```python
from build123d import *

# Parameters (mm, degrees)
F0_W     = 60
F0_H     = 60
F1_DEPTH = 32
F2_W     = 18
F2_H     = 20
F3_DEPTH = 60.001
F4_W     = 35
F4_H     = 10
F5_DEPTH = 60.001
F6_R     = 17.5
F6_R_2   = 10
F7_DEPTH = 64


with BuildPart() as f1:
    # F0 (on Top) → F1 (new body)
    with BuildSketch(Plane.XY):
        with Locations((0.728403, 0.219683)):
            Rectangle(F0_W, F0_H)
    extrude(amount=F1_DEPTH)

    # F2 (on face) → F3 (cut, through all)
    with BuildSketch(Plane.XZ.offset(29.780317)):
        with Locations((0.728403, 10)):
            Rectangle(F2_W, F2_H)
    extrude(amount=-F3_DEPTH, mode=Mode.SUBTRACT)

    # F4 (on face) → F5 (cut, through all)
    with BuildSketch(Plane.YZ.offset(30.728403)):
        with Locations((0.219683, 5)):
            Rectangle(F4_W, F4_H)
    extrude(amount=-F5_DEPTH, mode=Mode.SUBTRACT)

    # F6 (on face) → F7 (join)
    with BuildSketch(Plane.XY.offset(32)):
        Circle(F6_R)
        Circle(F6_R_2, mode=Mode.SUBTRACT)
    extrude(amount=F7_DEPTH)


solid = f1.part
```
Geometry: final body of the model. Coordinates: model frame, mm. A direction names the side the tool comes from. Coordinates: 2 decimals unless noted, no trailing zeros. Order: outer loops, then holes, each group sorted by start corner. A loop starts at its lowest first (then second) coordinate and runs counter-clockwise, first axis right, second up. Notation, with made-up numbers: (53.5, 85) -> (103.5, 85) arc R24 ccw to (103.5, 118) -> close; hole circle Ø3 at (-8.75, 22). An arc over 180 degrees is marked (long way). Use CSV: the item, a comma, the result in double quotes.
1) Access query for faces 5 (the flat face through (9.728, 0, 12)), 6 (the flat face through (0, 0, 32)), 7 (the flat face through (-19, 0, 10)), 8 (the flat face through (0, 30.22, 23)), 9 (the flat face through (30.728, 0, 19)). Directions: +Z, -Z, +X, -X, +Y, -Y. A direction counts if a zero-diameter tool reaches every point of the face in a straight line with its end or side. Return the directions, or none.
Findings:
face 5,"-Z, +Y, -Y"
face 6,"+Z"
face 7,"-Z, +X, -X"
face 8,"+Z, -Z, +X, -X, +Y"
face 9,"+Z, -Z, +X, +Y, -Y"
2) Section A-A on x = 0. Output: boundary loops of the cut face in (y, z).
Findings:
outline,"(-29.78, 20) -> (30.22, 20) -> (30.22, 32) -> (17.5, 32) -> (17.5, 96) -> (10, 96) -> (10, 32) -> (-10, 32) -> (-10, 96) -> (-17.5, 96) -> (-17.5, 32) -> (-29.78, 32) -> close"
3) Mould query, pull axis X, two halves, no side actions, for faces 1 (the flat face through (-29.272, 0, 19)), 2 (the cylindrical face through (-2.17, -9.76, 63.55)), 3 (the flat face through (-19, 24, 0)), 4 (the flat face through (1, 0, 20)). Classes: +X half, -X half, draft (parallel to the pull), parting line (faces both ways), or undercut.
Findings:
face 1,"-X half"
face 2,"undercut"
face 3,"draft"
face 4,"undercut"
4) Section C-C on z = 44.5. Output: boundary loops of the cut face in (x, y), then the cut area to 3 significant figures.
Findings:
outline,"circle Ø35 at (0, 0); hole circle Ø20 at (0, 0)"
area,"648 mm^2"
5) Line query: line 1 (Y direction, x = 0, z = 50); line 2 (X direction, y = -0.5, z = 11.5); line 3 (Z direction, x = -21, y = 13). Output: solid intervals per line, ascending.
Findings:
line 1,"y = -17.5 to -10, 10 to 17.5"
line 2,"x = -29.27 to -8.27, 9.73 to 30.73"
line 3,"z = 10 to 32"
6) Pin query (flat end, axial travel): pin 1 Ø5 at (x, z) = (-8, 40.5) entering from +Y; pin 2 Ø10.5 at (x, y) = (-22.5, -1.5) entering from -Z; pin 3 Ø3 at (x, y) = (-14.5, -23.5) entering from +Z. Return the tip coordinate at first contact, or that it passes through.
Findings:
pin 1,"stops at y = 16.61"
pin 2,"stops at z = 10"
pin 3,"stops at z = 32"
7) Section D-D on x = -20. Output: boundary loops of the cut face in (y, z).
Findings:
outline,"(-29.78, 0) -> (-17.28, 0) -> (-17.28, 10) -> (17.72, 10) -> (17.72, 0) -> (30.22, 0) -> (30.22, 32) -> (-29.78, 32) -> close"
8) Section B-B on y = 14. Output: boundary loops of the cut face in (x, z), then the cut area to 3 significant figures.
Findings:
outline,"(-29.27, 10) -> (-8.27, 10) -> (-8.27, 20) -> (9.73, 20) -> (9.73, 10) -> (30.73, 10) -> (30.73, 32) -> (10.5, 32) -> (10.5, 96) -> (-10.5, 96) -> (-10.5, 32) -> (-29.27, 32) -> close"
area,"2,480 mm^2"
